The figure shows three views and two pictorial views of one solid part (mm, origin at its lowest corner). Answer the questions. A direction names the side the tool comes from. Coordinates: 2 decimals unless noted, no trailing zeros. Write each loop counter-clockwise with the first axis right and the second up, starting at its lowest first coordinate (ties: lowest second). Pieces come first, ordered by that corner, then holes. Notation, with made-up numbers: (55.5, 49.5) - (94.5, 49.5) arc R19 cw to (94.5, 60.5) - close; hole circle Ø4 at (61.5, -23.75). An arc over 180 degrees is marked (long way). Use a Markdown table: item, result. Add a question column.
(1) For a pull along Z with two mould halves and no side action, classify the marked faces 3, 4, 5 and 6 as released by +Z, released by -Z, zero draft, split by the parting line, or undercut.
(2) Given pin 1 Ø1 at (x, y) = (5.5, 13.5) entering from +Z; pin 2 Ø10 at (x, y) = (7.5, 12) entering from +Z; pin 3 Ø2 at (y, z) = (17, 11.5) entering from -X, each flat-ended and moving along its own axis, determine where each tip first touches the part or whether it passes through.
(3) A tool of negligible diameter and unlimited length cuts with its end or side. For the marked faces 1 and 2, from which of +Z, -Z, +X, -X, +Y, -Y can it reach the whole face along a straight path? Write none if from no direction.
(4) The part is cut by section A-A, the plane z = 27.5. Give the vertices of the cut face in (x, y).
(5) The part is cut by section C-C, the plane z = 16. Give the vertices of the cut face in (x, y), then the cut area to 3 significant figures.
(6) The part is cut by section B-B, the plane x = 8.5. Give the vertices of the cut face in (y, z), then the cut area to 3 significant figures.
(7) The part is cut by section D-D, the plane y = 15. Give the vertices of the cut face in (x, z), then the cut area to 3 significant figures.
(8) Find the intervals of material crossed by line 1 (Z direction, x = 8.5, y = 2.5); line 2 (X direction, y = 1.2, z = 27.5); line 3 (Y direction, x = 8.5, z = 14), in increasing order. Write a range as from..to.
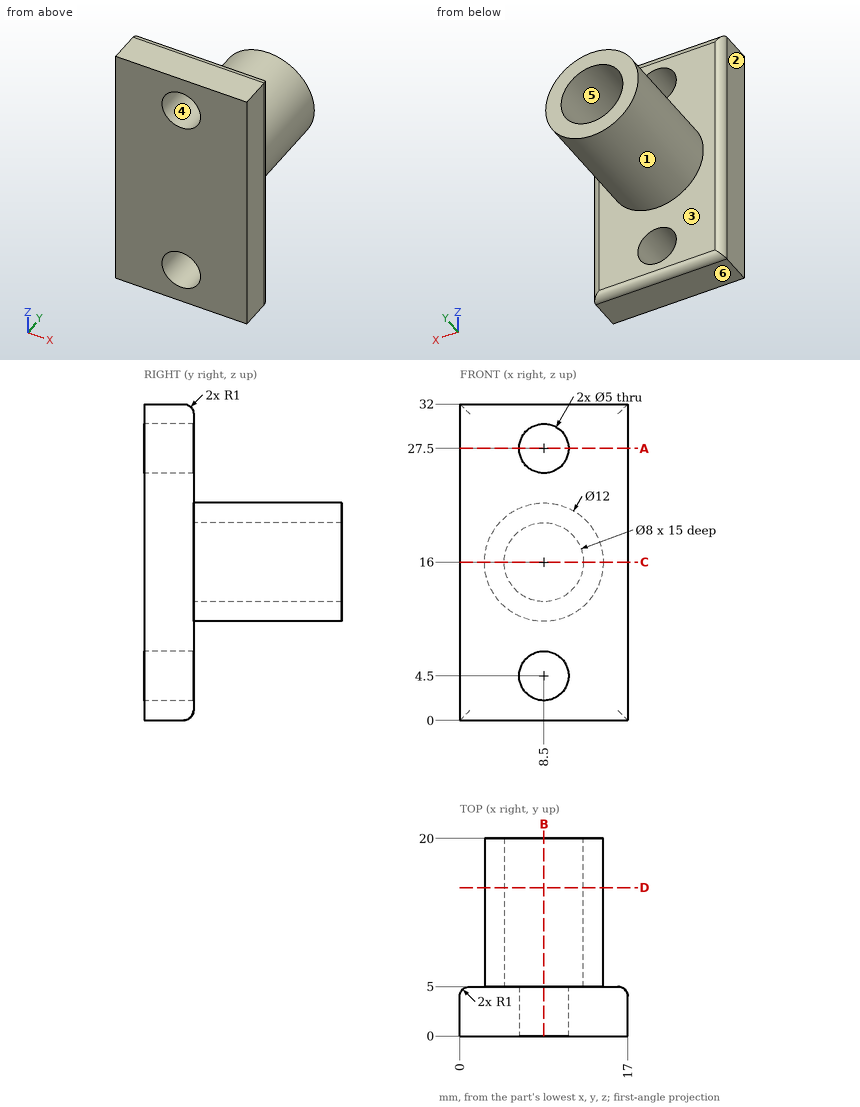
Model answer:
| question | item | result |
|---|---|---|
| 1 | face 3 | zero draft |
| 1 | face 4 | undercut |
| 1 | face 5 | undercut |
| 1 | face 6 | released by -Z |
| 2 | pin 1 | z = 21.45 |
| 2 | pin 2 | z = 22 |
| 2 | pin 3 | x = 3.63 |
| 3 | face 1 | +Y |
| 3 | face 2 | +Z, -Z, -X, +Y, -Y |
| 4 | outline | (0, 0) - (6, 0) - (6, 5) - (1, 5) arc R1 ccw to (0, 4) - close; (11, 0) - (17, 0) - (17, 4) arc R1 ccw to (16, 5) - (11, 5) - close |
| 5 | outline | (0, 0) - (17, 0) - (17, 4) arc R1 ccw to (16, 5) - (14.5, 5) - (14.5, 20) - (12.5, 20) - (12.5, 5) - (4.5, 5) - (4.5, 20) - (2.5, 20) - (2.5, 5) - (1, 5) arc R1 ccw to (0, 4) - close |
| 5 | area | 145 mm^2 |
| 6 | outline | (0, 0) - (4, 0) arc R1 ccw to (5, 1) - (5, 2) - (0, 2) - close; (0, 7) - (5, 7) - (5, 10) - (20, 10) - (20, 12) - (5, 12) - (5, 20) - (20, 20) - (20, 22) - (5, 22) - (5, 25) - (0, 25) - close; (0, 30) - (5, 30) - (5, 31) arc R1 ccw to (4, 32) - (0, 32) - close |
| 6 | area | 170 mm^2 |
| 7 | outline | circle Ø12 at (8.5, 16); hole circle Ø8 at (8.5, 16) |
| 7 | area | 62.8 mm^2 |
| 8 | line 1 | 0..2, 7..25, 30..32 |
| 8 | line 2 | 0..6, 11..17 |
| 8 | line 3 | 0..5 |
